Verification items for the finished model (mm, model axes). Face numbers are marked on the shaded views. A direction names the side the tool comes from. Coordinates: 2 decimals unless noted, no trailing zeros. Loops run counter-clockwise (first coordinate to the right, second up) from the corner with the lowest first, then second, coordinate; pieces in that order, holes last.
Q1. Sectioned sample at B-B (y = -17). Enter the section's corners in (x, z), then the cut area to 3 significant figures.
Q2. Sectioned sample at A-A (z = 0). Enter the section's corners in (x, y).
Q3. Material ranges on probe 1 along Z at (x, y) = (31.5, -3.5); probe 2 along Z at (x, y) = (-7, -16); probe 3 along X at (y, z) = (-23.75, -11.5), recorded low to high.
Q4. Sectioned sample at C-C (x = -16.5). Enter the section's corners in (y, z).
Q5. Go/stop test with flat-tipped pins: P1, Ø2.5, axis at y = -7, z = 11.5, coming from the +X side; P2, Ø8.5, axis at y = -21, z = -5, coming from the -X side; P3, Ø0.9, axis at x = 31.5, z = -11, coming from the +Y side. Record where each tip stops, or that it passes through.
Q6. Access from +Z, -Z, +X, -X, +Y, -Y to the whole of each face (thin tool, end or side, straight path). Record for the marked faces 1, 2 and 3.
Q7. Sectioned sample at D-D (x = -31.5). Enter the section's corners in (y, z), then the cut area to 3 significant figures.
Q8. Mould release check, pull along X, two halves, no side actions. Record for the marked faces 4, 5, 6 and 7: +X half, -X half, draft (parallel to the pull), parting line (faces both ways), or undercut.
```python
from build123d import *

# Parameters (mm, degrees)
F0_W      = 70
F0_H      = 30
F1_DEPTH  = 30
F2_T      = -2
F3_R      = 3
F3_W      = 12
F3_H      = 12
F3_W_2    = 24
F3_H_2    = 13
F4_DEPTH  = 30.001
F5_W      = 5
F5_H      = 5
F6_DEPTH  = 28
F7_R      = 1.5
F8_DEPTH  = 10
F9_W      = 10
F9_H      = 30
F10_DEPTH = 2
F12_R     = 1.5
F13_DEPTH = 30.001


with BuildPart() as f1:
    # F0 (on Front) → F1 (new body)
    with BuildSketch(Plane.XZ):
        Rectangle(F0_W, F0_H)
    extrude(amount=F1_DEPTH)

    # F2
    f2_openings = [f1.faces().sort_by_distance(p)[0] for p in [
        (0, 0, 0),
    ]]
    offset(amount=F2_T, openings=f2_openings)

    # F3 (on face) → F4 (cut, through all)
    with BuildSketch(Plane.XZ.offset(30)):
        with Locations((-27, 0)):
            Circle(F3_R)
        with Locations((23, 0)):
            Rectangle(F3_W, F3_H)
        with Locations((-8, 0)):
            Rectangle(F3_W_2, F3_H_2)
    extrude(amount=-F4_DEPTH, mode=Mode.SUBTRACT)

    # F5 (on face) → F6 (join, through all)
    with BuildSketch(Plane(origin=(0, 0, 0), x_dir=(-1, 0, 0), z_dir=(0, 1, 0))):
        with Locations((-30.5, 10.5)):
            Rectangle(F5_W, F5_H)
        with Locations((30.5, 10.5)):
            Rectangle(F5_W, F5_H)
        with Locations((30.5, -10.5)):
            Rectangle(F5_W, F5_H)
        with Locations((-30.5, -10.5)):
            Rectangle(F5_W, F5_H)
    extrude(amount=-F6_DEPTH)

    # F7 (on face) → F8 (cut)
    with BuildSketch(Plane(origin=(0, 0, 0), x_dir=(-1, 0, 0), z_dir=(0, 1, 0))):
        with Locations((-31.5, 11.5)):
            Circle(F7_R)
        with Locations((31.5, 11.5)):
            Circle(F7_R)
        with Locations((-31.5, -11.5)):
            Circle(F7_R)
        with Locations((31.5, -11.5)):
            Circle(F7_R)
    extrude(amount=-F8_DEPTH, mode=Mode.SUBTRACT)



with BuildPart() as f10:
    # F9 (on face) → F10 (new body)
    with BuildSketch(Plane.XY.offset(15)):
        with Locations((-40, -15)):
            Rectangle(F9_W, F9_H)
    extrude(amount=-F10_DEPTH)


with BuildPart() as f1_1:
    add(f1.part)

    add(f10.part)  # F11 merges F10
    # F11: F10 across plane
    add(f10.part.mirror(Plane.YZ))

    # F12 (on face) → F13 (cut, through all)
    with BuildSketch(Plane.XY.offset(15)):
        with Locations((-38.7428589165, -6.7958449945)):
            Circle(F12_R)
        with Locations((38.7428589165, -6.7958449945)):
            Circle(F12_R)
        with Locations((-38.7428589165, -23.2041550055)):
            Circle(F12_R)
        with Locations((38.7428589165, -23.2041550055)):
            Circle(F12_R)
    extrude(amount=-F13_DEPTH, mode=Mode.SUBTRACT)


solid = f1_1.part
```
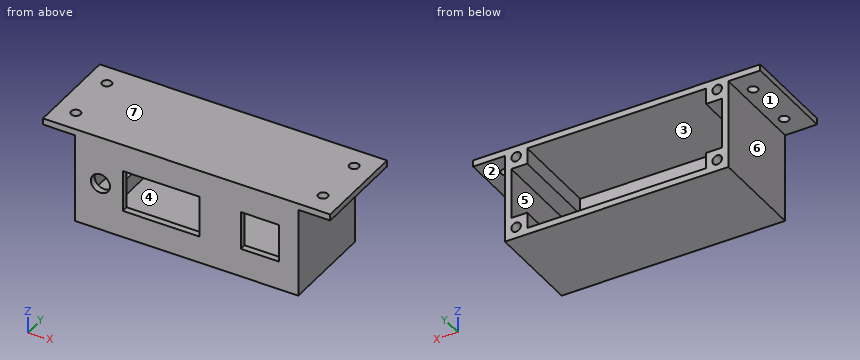
Geometry check:
1. outline: (-45, 13) - (-35, 13) - (-35, -15) - (35, -15) - (35, 13) - (45, 13) - (45, 15) - (-45, 15) - close; hole (-33, -8) - (-28, -8) - (-28, -13) - (28, -13) - (28, -8) - (33, -8) - (33, 8) - (28, 8) - (28, 13) - (-28, 13) - (-28, 8) - (-33, 8) - close
1. area: 524 mm2
2. outline: (-35, -30) - (-30, -30) - (-30, -28) - (-33, -28) - (-33, 0) - (-35, 0) - close; (-24, -30) - (-20, -30) - (-20, -28) - (-24, -28) - close; (4, -30) - (17, -30) - (17, -28) - (4, -28) - close; (29, -30) - (35, -30) - (35, 0) - (33, 0) - (33, -28) - (29, -28) - close
3. probe 1: z = -15 to -13, -10 to -8, 8 to 10, 13 to 15
3. probe 2: z = -15 to -13, 13 to 15
3. probe 3: x = -35 to -28, 28 to 35
4. outline: (-30, -15) - (0, -15) - (0, -13) - (-28, -13) - (-28, -6.5) - (-30, -6.5) - close; (-30, 6.5) - (-28, 6.5) - (-28, 13) - (0, 13) - (0, 15) - (-30, 15) - close
5. P1: stops at x = 35
5. P2: stops at x = -35
5. P3: stops at y = -10
6. face 1: -Z, -X, +Y, -Y
6. face 2: -Z, +X, +Y, -Y
6. face 3: +Y
7. outline: (-30, -15) - (0, -15) - (0, -13) - (-10, -13) - (-10, -10) - (0, -10) - (0, -8) - (-28, -8) - (-28, 8) - (0, 8) - (0, 10) - (-10, 10) - (-10, 13) - (0, 13) - (0, 15) - (-30, 15) - close
7. area: 392 mm2
8. face 4: undercut
8. face 5: undercut
8. face 6: -X half
8. face 7: draft
